Build history of the part. All positions in model axes, mm. Face numbers are marked on the shaded views. A direction names the side the tool comes from. Give positions to 0.01 mm unless a question says otherwise; leave off trailing zeros. Order: outer loops, then holes, each group sorted by start corner. A loop starts at its lowest first (then second) coordinate and runs counter-clockwise, first axis right, second up. Notation, with made-up numbers: M 61.5,0 L 114.5,0 A25 ccw 114.5,33 Z; hole C 86.5,63 d6. An arc over 180 degrees is marked long. One line per item, written item: value.
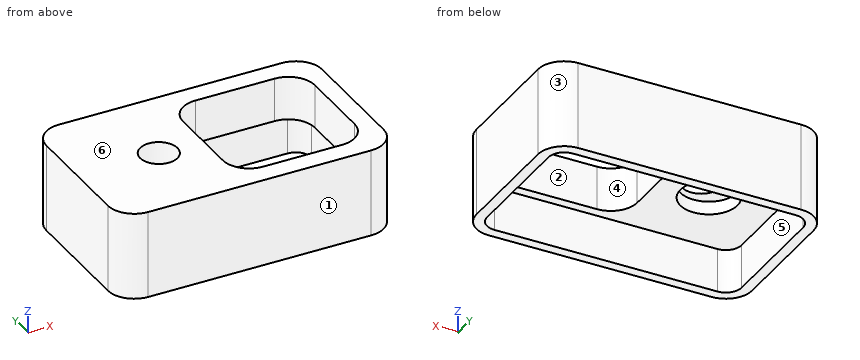
from build123d import *

# Parameters (mm, degrees)
SKETCH2_W           = 62.8
SKETCH2_H           = 38.3
SKETCH2_R           = 4.25
SKETCH2_W_2         = 30
SKETCH2_H_2         = 29
BOSS_EXTRUDE1_DEPTH = 10
SKETCH2_3_W         = 62.8
SKETCH2_3_H         = 38.3
SKETCH2_3_W_2       = 58
SKETCH2_3_H_2       = 33.5
BOSS_EXTRUDE2_DEPTH = 10
SKETCH2_4_R         = 6.5
CUT_EXTRUDE1_DEPTH  = 3
FILLET1_R           = 3.6
FILLET2_R           = 6


with BuildPart() as part:
    # Sketch2 → Boss-Extrude1 (new body)
    with BuildSketch(Plane.XY):
        with Locations((29, -16.75)):
            Rectangle(SKETCH2_W, SKETCH2_H)
        with Locations((16.2, -16.75)):
            Circle(SKETCH2_R, mode=Mode.SUBTRACT)
        with Locations((41.25, -16.75)):
            Rectangle(SKETCH2_W_2, SKETCH2_H_2, mode=Mode.SUBTRACT)
    extrude(amount=BOSS_EXTRUDE1_DEPTH)

    # Sketch2<3> → Boss-Extrude2 (add)
    with BuildSketch(Plane.XY):
        with Locations((29, -16.75)):
            Rectangle(SKETCH2_3_W, SKETCH2_3_H)
        with Locations((29, -16.75)):
            Rectangle(SKETCH2_3_W_2, SKETCH2_3_H_2, mode=Mode.SUBTRACT)
    extrude(amount=-BOSS_EXTRUDE2_DEPTH)

    # Sketch2<4> → Cut-Extrude1 (cut)
    with BuildSketch(Plane.XY):
        with Locations((14.45, -16.75)):
            Circle(SKETCH2_4_R)
    extrude(amount=CUT_EXTRUDE1_DEPTH, mode=Mode.SUBTRACT)

    # Fillet1
    fillet1_edges = [part.edges().sort_by_distance(p)[0] for p in [
        (58, 0, -5),
        (0, 0, -5),
        (0, -33.5, -5),
        (58, -33.5, -5),
    ]]
    fillet(fillet1_edges, radius=FILLET1_R)

    # Fillet2
    fillet2_edges = [part.edges().sort_by_distance(p)[0] for p in [
        (26.25, -2.25, 5),
        (26.25, -31.25, 5),
        (56.25, -31.25, 5),
        (56.25, -2.25, 5),
        (60.4, -35.9, 0),
        (-2.4, -35.9, 0),
        (-2.4, 2.4, 0),
        (60.4, 2.4, 0),
    ]]
    fillet(fillet2_edges, radius=FILLET2_R)


solid = part.part
1) Saw through at B-B, the plane x = 44. Write the cut outline in (y, z), then the cut area to 3 significant figures.
Check values:
outline: M -35.9,-10 L -33.5,-10 L -33.5,0 L -31.25,0 L -31.25,10 L -35.9,10 Z; M -2.25,0 L 0,0 L 0,-10 L 2.4,-10 L 2.4,10 L -2.25,10 Z
area: 141 mm^2
2) Saw through at C-C, the plane x = 23. Write the cut outline in (y, z).
Check values:
outline: M -35.9,-10 L -33.5,-10 L -33.5,0 L 0,0 L 0,-10 L 2.4,-10 L 2.4,10 L -35.9,10 Z
3) Saw through at A-A, the plane y = -16.75. Write the cut outline in (x, z), then the cut area to 4 significant figures.
Check values:
outline: M -2.4,-10 L 0,-10 L 0,0 L 7.95,0 L 7.95,3 L 11.95,3 L 11.95,10 L -2.4,10 Z; M 20.45,3 L 20.95,3 L 20.95,0 L 26.25,0 L 26.25,10 L 20.45,10 Z; M 56.25,0 L 58,0 L 58,-10 L 60.4,-10 L 60.4,10 L 56.25,10 Z
area: 277.5 mm^2
4) Drill centre lines: probe 1 along X at (y, z) = (-16.75, 5.75); probe 2 along Y at (x, z) = (16.2, 6); probe 3 along Y at (x, z) = (39, -6.75). Where is each one in solid material? Low to high. Write a range as from..to.
Check values:
probe 1: -2.4..11.95, 20.45..26.25, 56.25..60.4
probe 2: -35.9..-21, -12.5..2.4
probe 3: -35.9..-33.5, 0..2.4
5) Saw through at D-D, the plane y = -29. Write the cut outline in (x, z), then the cut area to 3 significant figures.
Check values:
outline: M -2.4,-10 L 0,-10 L 0,0 L 27.57,0 L 27.57,10 L -2.4,10 Z; M 54.93,0 L 58,0 L 58,-10 L 60.4,-10 L 60.4,10 L 54.93,10 Z
area: 402 mm^2
6) Tool access for the marked faces 4, 5 and 6: list every direction of +Z, -Z, +X, -X, +Y, -Y with a clear straight run to the whole face (end or side of a thin tool).
Check values:
face 4: +Z, -Z
face 5: -Z
face 6: +Z, +X, -X, +Y, -Y
7) Mould opens along Y. For the marked faces 1, 2 and 3 say: released by +Y, released by -Y, zero draft, split by the parting line, or undercut.
Check values:
face 1: released by -Y
face 2: undercut
face 3: released by +Y
8) Pin check, flat tips, straight feed: pin 1 (5 mm diameter, centred on x = 51, y = -5.5, fed in from -Z); pin 2 (6.5 mm diameter, centred on x = 12.5, y = -20, fed in from -Z). Stop position of each tip, or through.
Check values:
pin 1: through
pin 2: z = 0
